The listing builds one solid part. Answer for the finished solid, in the listing's coordinates (mm). Give positions to 0.01 mm unless a question says otherwise; leave off trailing zeros. Write each loop counter-clockwise with the first axis right and the second up, starting at its lowest first coordinate (ties: lowest second). Pieces come first, ordered by that corner, then holes. Notation, with made-up numbers: (83.25, -31.5) - (135.25, -31.5) arc R22 cw to (135.25, -9.5) - close; hole circle Ø1 at (65.25, 23). An arc over 180 degrees is marked (long way). Return JSON: item names as keys, results as strings.
from build123d import *

# Parameters (mm, degrees)
F0_W     = 177.8
F0_H     = 127
F0_R     = 38.1
F1_DEPTH = 25.4


with BuildPart() as f1:
    # F0 (on Front) → F1 (new body)
    with BuildSketch(Plane.XZ):
        with Locations((25.4, -53.399413)):
            Rectangle(F0_W, F0_H)
        with Locations((0, -53.399413)):
            Circle(F0_R, mode=Mode.SUBTRACT)
        Polygon((-63.5, 10.100587), (114.3, 10.100587), (-4.841213, 111.700587), align=None)
    extrude(amount=F1_DEPTH)


solid = f1.part
Item 1: A cutting plane is placed at B-B on x = -10. Determine the outline of the cut face in (y, z).
Answer below:
{"outline": "(-25.4, -116.9) - (0, -116.9) - (0, -90.16) - (-25.4, -90.16) - close; (-25.4, -16.64) - (0, -16.64) - (0, 102.77) - (-25.4, 102.77) - close"}
Item 2: A cutting plane is placed at D-D on x = 87.5. Determine the outline of the cut face in (y, z).
Answer below:
{"outline": "(-25.4, -116.9) - (0, -116.9) - (0, 32.95) - (-25.4, 32.95) - close"}
Item 3: A cutting plane is placed at C-C on y = -5.5. Determine the outline of the cut face in (x, z), then the cut area to 3 significant figures.
Answer below:
{"outline": "(-63.5, -116.9) - (114.3, -116.9) - (114.3, 10.1) - (-4.84, 111.7) - (-63.5, 10.1) - close; hole circle Ø76.2 at (0, -53.4)", "area": "27,100 mm²"}
Item 4: Consider L1, parallel to Z at x = 20, y = -4; L2, parallel to Z at x = 25, y = -16; L3, parallel to X at y = -20, z = -31.5. Determine where each line is inside the solid, lowest interval first.
Answer below:
{"L1": "z = -116.9 to -85.83, -20.97 to 90.52", "L2": "z = -116.9 to -82.15, -24.65 to 86.25", "L3": "x = -63.5 to -31.18, 31.18 to 114.3"}
Item 5: A cutting plane is placed at A-A on z = -47. Determine the outline of the cut face in (x, y), then the cut area to 3 significant figures.
Answer below:
{"outline": "(-63.5, -25.4) - (-37.56, -25.4) - (-37.56, 0) - (-63.5, 0) - close; (37.56, -25.4) - (114.3, -25.4) - (114.3, 0) - (37.56, 0) - close", "area": "2,610 mm²"}
Item 6: Flat-ended cylindrical pins translate along their axes: P1, Ø10, axis at x = 11.5, y = -17, coming from the +Z side; P2, Ø5, axis at x = 9, z = -19.5, coming from the -Y side; P3, Ø10, axis at y = -19, z = 27.5, coming from the +X side; P4, Ø5, axis at x = 56.5, y = -5, coming from the +Z side. Find the tip coordinate at first contact, or state that the pin passes through.
Answer below:
{"P1": "stops at z = 102.03", "P2": "passes through", "P3": "stops at x = 99.76", "P4": "stops at z = 61.52"}
Item 7: The mould has two halves that part along X. Classify faces 1 (the face through (-4.96, -12.522, -15.624)), 2 (the face through (55.56, -12.52, 60.19)), 3 (the face through (24, -13, -116.899)): +X half, -X half, draft (parallel to the pull), parting line (faces both ways), or undercut.
Answer below:
{"face 1": "undercut", "face 2": "+X half", "face 3": "draft"}
